Input: part model. Units: mm. Frame: model coordinates. A direction names the side the tool comes from. Give positions to 0.01 mm unless a question says otherwise; leave off trailing zeros. Write each loop counter-clockwise with the first axis right and the second up, starting at its lowest first coordinate (ties: lowest second). Pieces come first, ordered by that corner, then holes.
```python
from build123d import *

# Parameters (mm, degrees)
F0_R     = 6.35
F1_DEPTH = 132.08
F2_R     = 12.7
F3_DEPTH = 2.54
F4_W     = 19.05
F4_H     = 19.05
F5_DEPTH = 2.38125
F6_R     = 6.35
F7_DEPTH = 4.7625


with BuildPart() as f1:
    # F0 (on Top) → F1 (new body)
    with BuildSketch(Plane.XY):
        Circle(F0_R)
    extrude(amount=F1_DEPTH)

    # F2 (on face) → F3 (join)
    with BuildSketch(Plane.XY.offset(132.08)):
        Circle(F2_R)
    extrude(amount=F3_DEPTH)

    # F4 (on Front) → F5 (join, symmetric)
    with BuildSketch(Plane.XZ):
        with Locations((0, 144.145)):
            Rectangle(F4_W, F4_H)
    extrude(amount=F5_DEPTH, both=True)

    # F6 (on face) → F7 (cut)
    with BuildSketch(Plane.XZ.offset(2.38125)):
        with Locations((0, 144.145)):
            Circle(F6_R)
    extrude(amount=-F7_DEPTH, mode=Mode.SUBTRACT)


solid = f1.part
```
Q1. Section C-C, the plane z = 118. Return the cut outline in (x, y), then the cut area to 3 significant figures.
Q2. Section B-B, the plane y = 0. Return the cut outline in (x, z) (3 decimals).
Q3. Access query for faces 1 (the cylindrical face through (-1.38, -6.2, 65.12)), 2 (the flat face through (0, -2.381, 151)), 3 (the flat face through (-9.525, 0, 144)). Directions: +Z, -Z, +X, -X, +Y, -Y. A direction counts if a zero-diameter tool reaches every point of the face in a straight line with its end or side. Return the directions, or none.
Q4. Material intervals for line 1 along Z through (x, y) = (0, -0.4) (3 decimals); line 2 along Z through (x, y) = (-1.5, -6); line 3 along Z through (x, y) = (-2.5, 11), sorted ascending.
Q5. Pin query (flat end, axial travel): pin 1 (8 mm diameter, centred on x = -7.5, y = -5.5, fed in from -Z); pin 2 (5.5 mm diameter, centred on x = 3, z = 140.5, fed in from +Y); pin 3 (10 mm diameter, centred on x = 4.5, z = 112, fed in from -Y); pin 4 (10 mm diameter, centred on y = 1, z = 77, fed in from -X). Return the tip coordinate at first contact, or that it passes through.
Q6. Section A-A, the plane x = 0. Return the cut outline in (y, z) (3 decimals), then the cut area to 3 significant figures.
Solutions:
1. outline: circle Ø12.7 at (0, 0)
1. area: 127 mm2
2. outline: (-12.7, 132.08) - (-6.35, 132.08) - (-6.35, 0) - (6.35, 0) - (6.35, 132.08) - (12.7, 132.08) - (12.7, 134.62) - (9.525, 134.62) - (9.525, 153.67) - (-9.525, 153.67) - (-9.525, 134.62) - (-12.7, 134.62) - close; hole circle Ø12.7 at (0, 144.145)
3. face 1: -Z
3. face 2: +Z, +X, -X, -Y
3. face 3: +Z, -X, +Y, -Y
4. line 1: z = 0 to 137.795, 150.495 to 153.67
4. line 2: z = 0 to 134.62
4. line 3: z = 132.08 to 134.62
5. pin 1: stops at z = 0
5. pin 2: stops at y = 2.38
5. pin 3: stops at y = -6.35
5. pin 4: stops at x = -6.35
6. outline: (-12.7, 132.08) - (-6.35, 132.08) - (-6.35, 0) - (6.35, 0) - (6.35, 132.08) - (12.7, 132.08) - (12.7, 134.62) - (2.381, 134.62) - (2.381, 137.795) - (-2.381, 137.795) - (-2.381, 134.62) - (-12.7, 134.62) - close; (-2.381, 150.495) - (2.381, 150.495) - (2.381, 153.67) - (-2.381, 153.67) - close
6. area: 1,770 mm2
